The listing builds one solid part. Answer for the finished solid, in the listing's coordinates (mm). Face numbers are marked on the shaded views. A direction names the side the tool comes from. Coordinates: 2 decimals unless noted, no trailing zeros. Write each loop counter-clockwise with the first axis right and the second up, starting at its lowest first coordinate (ties: lowest second). Pieces come first, ordered by that corner, then holes.
from build123d import *

# Parameters (mm, degrees)
CYLINDER295_R     = 2
CYLINDER295_DEPTH = 20
CYLINDER294_R     = 2
CYLINDER294_DEPTH = 20
BOX385_W          = 2
BOX385_H          = 5
BOX385_DEPTH      = 2
BOX025_W          = 23
BOX025_H          = 5
BOX025_DEPTH      = 25
BOX026_W          = 51
BOX026_H          = 5
BOX026_DEPTH      = 10
BOX024_W          = 51
BOX024_H          = 5
BOX024_DEPTH      = 25
BOX384_W          = 2
BOX384_H          = 5
BOX384_DEPTH      = 2


with BuildPart() as cylinder295:
    # Cylinder295 → Cylinder295 (new body)
    with BuildSketch(Plane(origin=(-16, -88, 43), x_dir=(1, 0, 0), z_dir=(0, -1, 0))):
        Circle(CYLINDER295_R)
    extrude(amount=CYLINDER295_DEPTH)


with BuildPart() as fusion233:
    # Cylinder294 → Cylinder294 (new body)
    with BuildSketch(Plane(origin=(-53, -88, 43), x_dir=(1, 0, 0), z_dir=(0, -1, 0))):
        Circle(CYLINDER294_R)
    extrude(amount=CYLINDER294_DEPTH)

    # Fusion233: union Cylinder295
    add(cylinder295.part)


with BuildPart() as box385:
    # Box385 → Box385 (new body)
    with BuildSketch(Plane(origin=(-24, -93, 26), x_dir=(1, 0, 0), z_dir=(0, 0, 1))):
        with Locations((1, 2.5)):
            Rectangle(BOX385_W, BOX385_H)
    extrude(amount=BOX385_DEPTH)


with BuildPart() as box025:
    # Box025 → Box025 (new body)
    with BuildSketch(Plane(origin=(-37, -93, 16), x_dir=(1, 0, 0), z_dir=(0, 0, 1))):
        with Locations((11.5, 2.5)):
            Rectangle(BOX025_W, BOX025_H)
    extrude(amount=BOX025_DEPTH)


with BuildPart() as box026:
    # Box026 → Box026 (new body)
    with BuildSketch(Plane(origin=(-51, -90, 31), x_dir=(1, 0, 0), z_dir=(0, 0, 1))):
        with Locations((25.5, 2.5)):
            Rectangle(BOX026_W, BOX026_H)
    extrude(amount=BOX026_DEPTH)


with BuildPart() as cut268:
    # Box024 → Box024 (new body)
    with BuildSketch(Plane(origin=(-51, -93, 16), x_dir=(1, 0, 0), z_dir=(0, 0, 1))):
        with Locations((25.5, 2.5)):
            Rectangle(BOX024_W, BOX024_H)
    extrude(amount=BOX024_DEPTH)

    # Fusion223: union Box026
    add(box026.part)

    # Cut268: cut Box025
    add(box025.part, mode=Mode.SUBTRACT)


with BuildPart() as cut268_1:
    # Cut268 placement: moved
    add(cut268.part.moved(Location((-9, 0, 10))))


with BuildPart() as cut280:
    # Box384 → Box384 (new body)
    with BuildSketch(Plane(origin=(-47, -93, 26), x_dir=(1, 0, 0), z_dir=(0, 0, 1))):
        with Locations((1, 2.5)):
            Rectangle(BOX384_W, BOX384_H)
    extrude(amount=BOX384_DEPTH)

    # Fusion224: union Box385, Cut268
    add(box385.part)
    add(cut268_1.part)


with BuildPart() as cut280_1:
    # Fusion224 placement: moved
    add(cut280.part.moved(Location((0, -5, -4))))

    # Cut280: cut Fusion233
    add(fusion233.part, mode=Mode.SUBTRACT)


solid = cut280_1.part
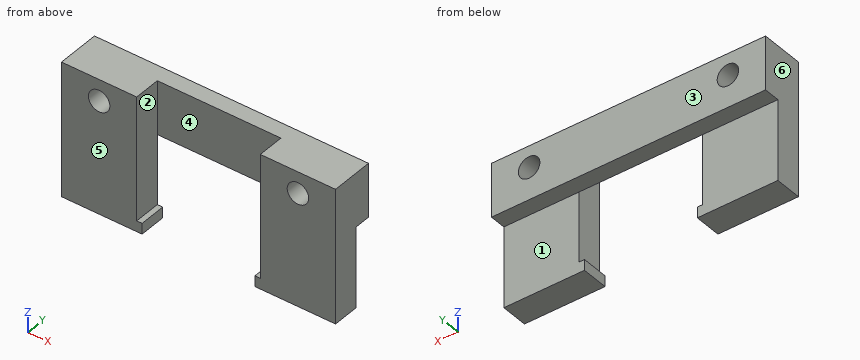
1. Find the intervals of material crossed by L1, parallel to X at y = -92.75, z = 43; L2, parallel to X at y = -96.5, z = 43; L3, parallel to X at y = -94.75, z = 26.75, in increasing order.
Results found:
L1: x = -60 to -55, -51 to -18, -14 to -9
L2: x = -60 to -55, -51 to -46, -23 to -18, -14 to -9
L3: x = -60 to -46, -23 to -9
2. Section D-D on z = 25.5 is taken. Give the vertices of the cut face in (x, y).
Results found:
outline: (-60, -98) - (-46, -98) - (-46, -93) - (-60, -93) - close; (-23, -98) - (-9, -98) - (-9, -93) - (-23, -93) - close
3. For a pull along X with two mould halves and no side action, classify the marked faces 4, 5 and 6 as pulls with the +X half, pulls with the -X half, needs draft (parallel to the pull), parting line crosses it, or undercut.
Results found:
face 4: undercut
face 5: needs draft
face 6: pulls with the -X half
4. Section C-C on z = 43 is taken. Give the vertices of the cut face in (x, y), then the cut area to 3 significant figures.
Results found:
outline: (-60, -98) - (-55, -98) - (-55, -90) - (-60, -90) - close; (-51, -98) - (-46, -98) - (-46, -93) - (-23, -93) - (-23, -98) - (-18, -98) - (-18, -90) - (-51, -90) - close; (-14, -98) - (-9, -98) - (-9, -90) - (-14, -90) - close
area: 229 mm2
5. Section A-A on y = -96 is taken. Give the vertices of the cut face in (x, z), then the cut area to 3 significant figures.
Results found:
outline: (-60, 22) - (-45, 22) - (-45, 24) - (-46, 24) - (-46, 47) - (-60, 47) - close; (-24, 22) - (-9, 22) - (-9, 47) - (-23, 47) - (-23, 24) - (-24, 24) - close; hole circle Ø4 at (-53, 43); hole circle Ø4 at (-16, 43)
area: 679 mm2
6. Section B-B on x = -16 is taken. Give the vertices of the cut face in (y, z).
Results found:
outline: (-98, 22) - (-93, 22) - (-93, 37) - (-90, 37) - (-90, 41) - (-98, 41) - close; (-98, 45) - (-90, 45) - (-90, 47) - (-98, 47) - close
7. A tool of negligible diameter and unlimited length cuts with its end or side. For the marked faces 1, 2 and 3, from which of +Z, -Z, +X, -X, +Y, -Y can it reach the whole face along a straight path? Write none if from no direction.
Results found:
face 1: -Z, +X, -X, +Y
face 2: +Z, -Y
face 3: +Z, -Z, +X, -X, +Y
8. Flat-ended cylindrical pins translate along their axes: P1, Ø4.5, axis at x = -49, z = 30, coming from the +Y side; P2, Ø0.8, axis at x = -45.5, y = -96.5, coming from the +Z side; P3, Ø3.5, axis at x = -46.5, y = -91.5, coming from the -Z side; P4, Ø2, axis at x = -34.5, y = -92.5, coming from the -Z side. Find the tip coordinate at first contact, or state that the pin passes through.
Results found:
P1: stops at y = -93
P2: stops at z = 24
P3: stops at z = 22
P4: stops at z = 37
